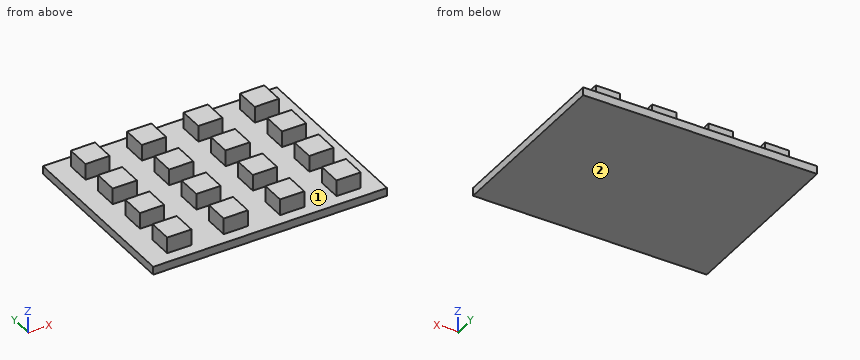
from build123d import *

# Parameters (mm, degrees)
F0_W     = 58
F0_H     = 45
F1_DEPTH = 2
F2_W     = 6
F2_H     = 6
F3_DEPTH = 4


with BuildPart() as f1:
    # F0 (on Top) → F1 (new body)
    with BuildSketch(Plane.XY):
        Rectangle(F0_W, F0_H)
    extrude(amount=F1_DEPTH)

    # F2 (on face) → F3 (join)
    with BuildSketch(Plane.XY.offset(2)):
        with Locations((-21, 16.386651)):
            Rectangle(F2_W, F2_H)
        with Locations((-7, 16.386651)):
            Rectangle(F2_W, F2_H)
        with Locations((7, 16.386651)):
            Rectangle(F2_W, F2_H)
        with Locations((21, 16.386651)):
            Rectangle(F2_W, F2_H)
        with Locations((-20.923837, 5.386915)):
            Rectangle(F2_W, F2_H)
        with Locations((-6.923837, 5.386915)):
            Rectangle(F2_W, F2_H)
        with Locations((7.076163, 5.386915)):
            Rectangle(F2_W, F2_H)
        with Locations((21.076163, 5.386915)):
            Rectangle(F2_W, F2_H)
        with Locations((-20.847673, -5.612822)):
            Rectangle(F2_W, F2_H)
        with Locations((-6.847673, -5.612822)):
            Rectangle(F2_W, F2_H)
        with Locations((7.152327, -5.612822)):
            Rectangle(F2_W, F2_H)
        with Locations((21.152327, -5.612822)):
            Rectangle(F2_W, F2_H)
        with Locations((-20.77151, -16.612558)):
            Rectangle(F2_W, F2_H)
        with Locations((-6.77151, -16.612558)):
            Rectangle(F2_W, F2_H)
        with Locations((7.22849, -16.612558)):
            Rectangle(F2_W, F2_H)
        with Locations((21.22849, -16.612558)):
            Rectangle(F2_W, F2_H)
    extrude(amount=F3_DEPTH)


solid = f1.part
Verification items for the finished model (mm, model axes). Face numbers are marked on the shaded views. Round coordinates to 2 decimals unless told otherwise and drop trailing zeros. Loops run counter-clockwise (first coordinate to the right, second up) from the corner with the lowest first, then second, coordinate; pieces in that order, holes last. Notation, with made-up numbers: (-28.5, 52.25) - (3.5, 52.25) arc R21 cw to (3.5, 71.25) - close; hole circle Ø5 at (35, -33.5). An arc over 180 degrees is marked (long way). Use a Markdown table: item, result. Add a question column.
1. Section check D-D, the plane x = -14.5. Record the boundary of the cut face in (y, z), plus the area to 3 significant figures.
2. Section check A-A, the plane x = -7. Record the boundary of the cut face in (y, z).
3. Release check for a two-part mould opening along Y. For the marked faces 1 and 2 record: released by +Y, released by -Y, zero draft, split by the parting line, or undercut.
4. Thickness scan on probe 1 along Y at (x, z) = (-5.5, 3.75); probe 2 along X at (y, z) = (7.5, 4.4); probe 3 along Z at (x, y) = (-1.5, 19). Record the ranges inside material, lowest first. Write a range as [from, to].
5. Section check B-B, the plane z = 3.4. Give the number of separate pieces and of enclosed holes in the cut face, plus the area to 3 significant figures.
6. Section check C-C, the plane y = 7. Record the boundary of the cut face in (x, z), plus the area to 3 significant figures.
7. Gauge pin test, flat ends, axial feed: pin 1 (2 mm diameter, centred on x = 21, z = 4.5, fed in from +Y); pin 2 (2 mm diameter, centred on x = 6.5, z = 4, fed in from -Y); pin 3 (1.2 mm diameter, centred on y = -6, z = 4, fed in from +X). Record the tip position at first contact, or that the pin passes through.
Checks:
| question | item | result |
|---|---|---|
| 1 | outline | (-22.5, 0) - (22.5, 0) - (22.5, 2) - (-22.5, 2) - close |
| 1 | area | 90.0 mm^2 |
| 2 | outline | (-22.5, 0) - (22.5, 0) - (22.5, 2) - (19.39, 2) - (19.39, 6) - (13.39, 6) - (13.39, 2) - (8.39, 2) - (8.39, 6) - (2.39, 6) - (2.39, 2) - (-2.61, 2) - (-2.61, 6) - (-8.61, 6) - (-8.61, 2) - (-13.61, 2) - (-13.61, 6) - (-19.61, 6) - (-19.61, 2) - (-22.5, 2) - close |
| 3 | face 1 | undercut |
| 3 | face 2 | zero draft |
| 4 | probe 1 | y = [-19.61, -13.61], [-8.61, -2.61], [2.39, 8.39], [13.39, 19.39] |
| 4 | probe 2 | x = [-23.92, -17.92], [-9.92, -3.92], [4.08, 10.08], [18.08, 24.08] |
| 4 | probe 3 | z = [0, 2] |
| 5 | separate pieces | 16 |
| 5 | enclosed holes | 0 |
| 5 | area | 576 mm^2 |
| 6 | outline | (-29, 0) - (29, 0) - (29, 2) - (24.08, 2) - (24.08, 6) - (18.08, 6) - (18.08, 2) - (10.08, 2) - (10.08, 6) - (4.08, 6) - (4.08, 2) - (-3.92, 2) - (-3.92, 6) - (-9.92, 6) - (-9.92, 2) - (-17.92, 2) - (-17.92, 6) - (-23.92, 6) - (-23.92, 2) - (-29, 2) - close |
| 6 | area | 212 mm^2 |
| 7 | pin 1 | stops at y = 19.39 |
| 7 | pin 2 | stops at y = -19.61 |
| 7 | pin 3 | stops at x = 24.15 |
